```python
from build123d import *

# Parameters (mm, degrees)
SKETCH2_R               = 32.5
BOSS_EXTRUDE1_DEPTH     = 15
SKETCH3_R               = 27.5
CUT_EXTRUDE1_DEPTH      = 3
CUT_EXTRUDE2_START      = -12
SKETCH3_2_R             = 27.5
CUT_EXTRUDE2_DEPTH      = 3
CUT_EXTRUDE3_DEPTH      = 48.502631506
CUT_EXTRUDE3_DEPTH_BACK = 48.502631506
SKETCH4_R               = 8
SKETCH5_R               = 7.273402988
BOSS_EXTRUDE2_DEPTH     = 4.5
FILLET3_R               = 0.5
CUT_EXTRUDE4_DEPTH      = 49.833902158
CUT_EXTRUDE4_DEPTH_BACK = 49.833902158
SKETCH6_R               = 3


with BuildPart() as part:
    # Sketch2 → Boss-Extrude1 (new body)
    with BuildSketch(Plane(origin=(0, 0, 0), x_dir=(1, 0, 0), z_dir=(0, 1, 0))):
        with Locations(Location((0, 0, 0), (0, 0, 270))):
            Circle(SKETCH2_R)
    extrude(amount=BOSS_EXTRUDE1_DEPTH)

    # Sketch3 → Cut-Extrude1 (cut)
    with BuildSketch(Plane(origin=(0, 15, 0), x_dir=(1, 0, 0), z_dir=(0, 1, 0))):
        with Locations(Location((0, 0, 0), (0, 0, 270))):
            Circle(SKETCH3_R)
    extrude(amount=-CUT_EXTRUDE1_DEPTH, mode=Mode.SUBTRACT)

    # Sketch3_2 → Cut-Extrude2 (cut)
    with BuildSketch(Plane(origin=(0, 15, 0), x_dir=(1, 0, 0), z_dir=(0, 1, 0)).offset(CUT_EXTRUDE2_START)):
        with Locations(Location((0, 0, 0), (0, 0, 270))):
            Circle(SKETCH3_2_R)
    extrude(amount=-CUT_EXTRUDE2_DEPTH, mode=Mode.SUBTRACT)

    # Sketch4 → Cut-Extrude3 (cut, two sides: drawn at the far end of the back side and taken through both)
    with BuildSketch(Plane.XZ.offset(-3).offset(-CUT_EXTRUDE3_DEPTH_BACK)):
        with Locations(Location((0, 18, 0), (0, 0, 90))):
            Circle(SKETCH4_R)
        with Locations(Location((17.119017293, 5.562305899, 0), (0, 0, 90))):
            Circle(SKETCH4_R)
        with Locations(Location((10.580134541, -14.562305899, 0), (0, 0, 90))):
            Circle(SKETCH4_R)
        with Locations(Location((-10.580134541, -14.562305899, 0), (0, 0, 90))):
            Circle(SKETCH4_R)
        with Locations(Location((-17.119017293, 5.562305899, 0), (0, 0, 90))):
            Circle(SKETCH4_R)
    extrude(amount=CUT_EXTRUDE3_DEPTH + CUT_EXTRUDE3_DEPTH_BACK, mode=Mode.SUBTRACT)

    # Sketch5 → Boss-Extrude2 (add)
    with BuildSketch(Plane.XZ.offset(-3)):
        with Locations(Location((0, 0, 0), (0, 0, 90))):
            Circle(SKETCH5_R)
    extrude(amount=BOSS_EXTRUDE2_DEPTH)

    # Fillet3
    fillet3_edges = [part.edges().sort_by_distance(p)[0] for p in [
        (0, -1.5, -7.273402988),
    ]]
    fillet(fillet3_edges, radius=FILLET3_R)

    # Sketch6 → Cut-Extrude4 (cut, two sides: drawn at the far end of the back side and taken through both)
    with BuildSketch(Plane.XZ.offset(1.5).offset(-CUT_EXTRUDE4_DEPTH_BACK)):
        with Locations(Location((0, 0, 0), (0, 0, 270))):
            Circle(SKETCH6_R)
    extrude(amount=CUT_EXTRUDE4_DEPTH + CUT_EXTRUDE4_DEPTH_BACK, mode=Mode.SUBTRACT)


solid = part.part
```
CAD build for the part. Positions are in the model's coordinates, mm. A direction names the side the tool comes from. Give positions to 0.01 mm unless a question says otherwise; leave off trailing zeros. Loops run counter-clockwise (first coordinate to the right, second up) from the corner with the lowest first, then second, coordinate; pieces in that order, holes last. Notation, with made-up numbers: (70, 70) - (98, 70) arc R14 cw to (98, 79) - close; hole circle Ø10 at (0, 22.25). An arc over 180 degrees is marked (long way). Put each result on its own line as item: value.
Q1. Flat gauge pins, fed straight in: pin 1 (3 mm diameter, centred on x = 9, z = -22.5, fed in from -Y); pin 2 (7 mm diameter, centred on x = 0, z = 0, fed in from +Y); pin 3 (6 mm diameter, centred on y = 12, z = 19.5, fed in from +X); pin 4 (9.5 mm diameter, centred on x = 0, z = 18, fed in from +Y). Where does each tip first touch, or does it go through?
Filled in:
pin 1: stops at y = 3
pin 2: stops at y = 12
pin 3: stops at x = 28
pin 4: passes through
Q2. Mould opens along Z. For faces 4 (the face through (9.76, 7.4, 31)), 5 (the face through (-6, 12, 0)), 6 (the face through (7, 15, -27)) say: pulls with the +Z half, pulls with the -Z half, needs draft (parallel to the pull), parting line crosses it, or undercut.
Filled in:
face 4: parting line crosses it
face 5: undercut
face 6: needs draft
Q3. Tool access for faces 1 (the face through (0.9, 5.34, -2.86)), 2 (the face through (-24.397, 1.521, 12.69)), 3 (the face through (-24.397, 13.521, 12.69)): list every direction of +Z, -Z, +X, -X, +Y, -Y with a clear straight run to the whole face (end or side of a thin tool).
Filled in:
face 1: +Y, -Y
face 2: -Y
face 3: +Y
Q4. Slice it at A-A (x = 0). Give the cut face in (y, z), plus the area to 3 significant figures.
Filled in:
outline: (-1.5, -6.77) arc R0.5 ccw to (-1, -7.27) - (3, -7.27) - (3, -27.5) - (0, -27.5) - (0, -32.5) - (15, -32.5) - (15, -27.5) - (12, -27.5) - (12, -3) - (-1.5, -3) - close; (-1.5, 3) - (12, 3) - (12, 10) - (3, 10) - (3, 7.27) - (-1, 7.27) arc R0.5 ccw to (-1.5, 6.77) - close; (0, 27.5) - (3, 27.5) - (3, 26) - (12, 26) - (12, 27.5) - (15, 27.5) - (15, 32.5) - (0, 32.5) - close
area: 485 mm²
Q5. Slice it at B-B (z = 18). Give the cut face in (x, y), plus the area to 3 significant figures.
Filled in:
outline: (-27.06, 0) - (-20.79, 0) - (-20.79, 3) - (-8, 3) - (-8, 12) - (-20.79, 12) - (-20.79, 15) - (-27.06, 15) - close; (8, 3) - (20.79, 3) - (20.79, 0) - (27.06, 0) - (27.06, 15) - (20.79, 15) - (20.79, 12) - (8, 12) - close
area: 418 mm²
Q6. Slice it at D-D (z = 0). Give the number of separate pieces and of enclosed holes in the cut face, plus the area to 3 significant figures.
Filled in:
separate pieces: 4
enclosed holes: 0
area: 422 mm²
Q7. Probe line 1 along X through (y, z) = (1.5, 0); line 2 along X through (y, z) = (9.75, -16); line 3 along X through (y, z) = (9.5, -13). List the from-to ranges inside material, lowest first.
Filled in:
line 1: x = -32.5 to -27.5, -7.27 to -3, 3 to 7.27, 27.5 to 32.5
line 2: x = -28.29 to -18.45, -2.71 to 2.71, 18.45 to 28.29
line 3: x = -29.79 to -18.43, -2.73 to 2.73, 18.43 to 29.79
Q8. Slice it at C-C (y = 6). Give the cut face in (x, z), plus the area to 3 significant figures.
Filled in:
outline: circle Ø65 at (0, 0); hole circle Ø16 at (-17.12, 5.56); hole circle Ø16 at (-10.58, -14.56); hole circle Ø16 at (0, 18); hole circle Ø6 at (0, 0); hole circle Ø16 at (10.58, -14.56); hole circle Ø16 at (17.12, 5.56)
area: 2,280 mm²
